Source: CAD feature listing. Evaluate the final solid. Frame: model axes, mm. Face numbers are marked on the shaded views. Give positions to 0.01 mm unless a question says otherwise; leave off trailing zeros. Loops run counter-clockwise (first coordinate to the right, second up) from the corner with the lowest first, then second, coordinate; pieces in that order, holes last. Notation, with made-up numbers: M -28,83 L 27,83 A29 ccw 27,108 Z; hole C -17,30 d10. An arc over 180 degrees is marked long. Answer in a Markdown table with one row per item.
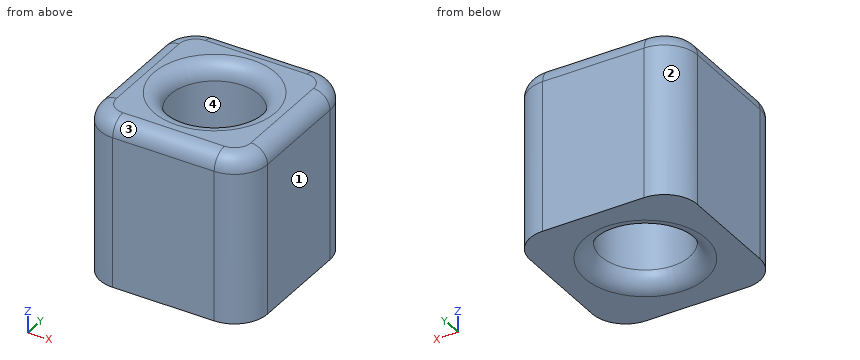
```python
from build123d import *

# Parameters (mm, degrees)
F0_W     = 50.8
F0_H     = 50.8
F1_DEPTH = 50.8
F2_R     = 13.4529093532
F3_DEPTH = 50.801
F4_R     = 10
F5_R     = 5


with BuildPart() as f1:
    # F0 (on Top) → F1 (new body)
    with BuildSketch(Plane.XY):
        with Locations((25.4, 25.4)):
            Rectangle(F0_W, F0_H)
    extrude(amount=F1_DEPTH)

    # F2 (on face) → F3 (cut, through all)
    with BuildSketch(Plane.XY.offset(50.8)):
        with Locations((25.1163877547, 25.6836116314)):
            Circle(F2_R)
    extrude(amount=-F3_DEPTH, mode=Mode.SUBTRACT)

    # F4
    f4_edges = [f1.edges().sort_by_distance(p)[0] for p in [
        (50.8, 50.8, 25.4),
        (50.8, 0, 25.4),
        (0, 50.8, 25.4),
        (0, 0, 25.4),
    ]]
    fillet(f4_edges, radius=F4_R)

    # F5
    f5_edges = [f1.edges().sort_by_distance(p)[0] for p in [
        (11.663478, 25.683612, 50.8),
        (11.663478, 25.683612, 0),
        (0, 25.4, 50.8),
        (2.928932, 47.871068, 50.8),
        (2.928932, 2.928932, 50.8),
        (25.4, 50.8, 50.8),
        (25.4, 0, 50.8),
        (47.871068, 47.871068, 50.8),
        (47.871068, 2.928932, 50.8),
        (50.8, 25.4, 50.8),
    ]]
    fillet(f5_edges, radius=F5_R)


solid = f1.part
```
Q1. Mould query, pull axis Y, two halves, no side actions, for the marked faces 1, 2, 3 and 4. Classes: +Y half, -Y half, draft (parallel to the pull), parting line (faces both ways), or undercut.
Values follow:
| item | result |
|---|---|
| face 1 | draft |
| face 2 | +Y half |
| face 3 | -Y half |
| face 4 | undercut |
Q2. Ray query, probe 1 along Y at (x, z) = (36.5, 21); probe 2 along X at (y, z) = (22.5, 8.5); probe 3 along Y at (x, z) = (26, 7.5). Return the intervals inside material, ascending. Write a range as from..to.
Values follow:
| item | result |
|---|---|
| probe 1 | 0..18.51, 32.85..50.8 |
| probe 2 | 0..12.05, 38.19..50.8 |
| probe 3 | 0..12.26, 39.11..50.8 |
Q3. Section query A-A (z = 36.5). Output: boundary loops of the cut face in (x, y), plus the area to 3 significant figures.
Values follow:
| item | result |
|---|---|
| outline | M 0,10 A10 ccw 10,0 L 40.8,0 A10 ccw 50.8,10 L 50.8,40.8 A10 ccw 40.8,50.8 L 10,50.8 A10 ccw 0,40.8 Z; hole C 25.12,25.68 d26.91 |
| area | 1,930 mm^2 |
Q4. Contact query for a flat-ended pin moving along its axis: pin 1 Ø3 at (y, z) = (5, 44) entering from +X. Output: stop coordinate, or through.
Values follow:
| item | result |
|---|---|
| pin 1 | x = 50.17 |
